Part print with two shaded views. Sizes in mm from the minimum x, y, z corner. Round coordinates to 2 decimals unless told otherwise and drop trailing zeros. Order: outer loops, then holes, each group sorted by start corner. A loop starts at its lowest first (then second) coordinate and runs counter-clockwise, first axis right, second up. Notation, with made-up numbers: M 1,54.5 L 40,54.5 A8 ccw 40,62.5 Z; hole C 71.25,-1 d9. An arc over 180 degrees is marked long. One line per question, with ' | ' between items.
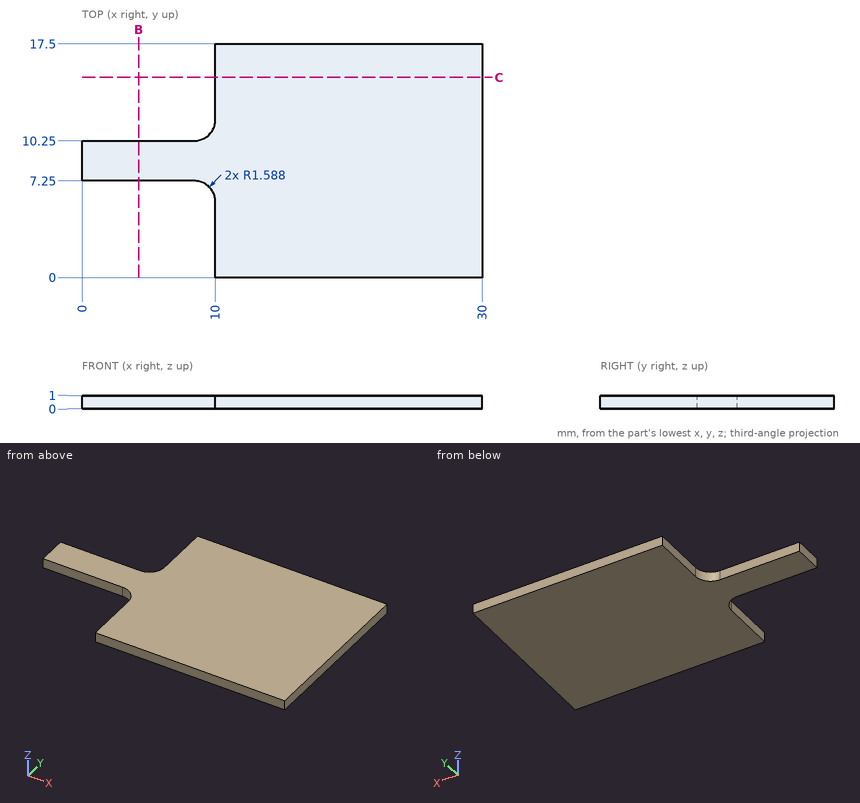
1) Probe line 1 (X direction, y = 13.25, z = 0.85); line 2 (Y direction, x = 1.5, z = 0.75); line 3 (Y direction, x = 8.75, z = 0.65) (1 decimal). List the from-to ranges inside material, lowest first. Write a range as [from, to].
The answers:
line 1: x = [10, 30] | line 2: y = [7.25, 10.25] | line 3: y = [7.2, 10.3]
2) Saw through at C-C (y = 15). List the corners of the cut face in (x, z).
The answers:
outline: M 10,0 L 30,0 L 30,1 L 10,1 Z
3) Saw through at B-B (x = 4.25). List the corners of the cut face in (y, z).
The answers:
outline: M 7.25,0 L 10.25,0 L 10.25,1 L 7.25,1 Z
